```python
from build123d import *

# Parameters (mm, degrees)
BOSS_EXTRUDE1_DEPTH = 300
SKETCH3_R           = 17
SKETCH3_R_2         = 30
CUT_EXTRUDE1_DEPTH  = 1055.907875982
SKETCH4_R           = 90
CUT_EXTRUDE2_DEPTH  = 20
SKETCH5_R           = 17
CUT_EXTRUDE3_DEPTH  = 1051
CHAMFER1_SIZE       = 70
CHAMFER1_SIZE2      = 120
FILLET1_R           = 20


with BuildPart() as part:
    # Sketch2 → Boss-Extrude1 (new body)
    with BuildSketch(Plane(origin=(0, 0, 0), x_dir=(-1, 0, 0), z_dir=(0, 1, 0))):
        Polygon((0, 0), (673.85334868, 0), (673.85334868, 900), (450, 900), (450, 145.843324447), (0, 145.843324447), align=None)
    extrude(amount=BOSS_EXTRUDE1_DEPTH)

    # Sketch3 → Cut-Extrude1 (cut, through all)
    with BuildSketch(Plane.XY.offset(145.843324447)):
        with Locations((-335, 150)):
            Circle(SKETCH3_R)
        with Locations((-228.822978678, 259.933547355)):
            Circle(SKETCH3_R)
        with Locations((-115, 150)):
            Circle(SKETCH3_R)
        with Locations((-225, 40)):
            Circle(SKETCH3_R)
        with Locations((-225, 150)):
            Circle(SKETCH3_R_2)
    extrude(amount=-CUT_EXTRUDE1_DEPTH, mode=Mode.SUBTRACT)

    # Sketch4 → Cut-Extrude2 (cut)
    with BuildSketch(Plane.XY.offset(145.843324447)):
        with Locations((-225, 150)):
            Circle(SKETCH4_R)
    extrude(amount=-CUT_EXTRUDE2_DEPTH, mode=Mode.SUBTRACT)

    # Sketch5 → Cut-Extrude3 (cut, through all)
    with BuildSketch(Plane.YZ.offset(-450)):
        with Locations(Location((75, 713.5, 0), (0, 0, 270))):
            Circle(SKETCH5_R)
        with Locations(Location((225, 713.5, 0), (0, 0, 270))):
            Circle(SKETCH5_R)
        with Locations(Location((75, 332.343324447, 0), (0, 0, 270))):
            Circle(SKETCH5_R)
        with Locations(Location((225, 332.343324447, 0), (0, 0, 270))):
            Circle(SKETCH5_R)
    extrude(amount=-CUT_EXTRUDE3_DEPTH, mode=Mode.SUBTRACT)

    # Chamfer1
    chamfer1_edges = [part.edges().sort_by_distance(p)[0] for p in [
        (-450, 150, 145.843324447),
    ]]
    chamfer1_side = [part.faces().sort_by_distance(p)[0] for p in [
        (-444.591673087, 150, 145.843324447),
    ]]
    chamfer(chamfer1_edges, length=CHAMFER1_SIZE, length2=CHAMFER1_SIZE2, reference=chamfer1_side[0])

    # Fillet1
    fillet1_edges = [part.edges().sort_by_distance(p)[0] for p in [
        (-380, 150, 145.843324447),
        (-450, 150, 265.843324447),
    ]]
    fillet(fillet1_edges, radius=FILLET1_R)


solid = part.part
```
Check sheet for the modelled part. Datum: model origin and axes. Units: mm. A direction names the side the tool comes from. Coordinates: 2 decimals unless noted, no trailing zeros. Loops run counter-clockwise (first coordinate to the right, second up) from the corner with the lowest first, then second, coordinate; pieces in that order, holes last.
1) Sectioned sample at A-A (y = 150). Record the boundary of the cut face in (x, z), and give its area (3 significant figures).
2) Gauge pin test, flat ends, axial feed: pin 1 (8 mm diameter, centred on y = 111, z = 159.5, fed in from +X); pin 2 (20.5 mm diameter, centred on y = 75, z = 332.34, fed in from +X); pin 3 (1.5 mm diameter, centred on y = 185.5, z = 650, fed in from +X). Record the tip position at first contact, or that the pin passes through.
3) Sectioned sample at B-B (x = -335). Record the boundary of the cut face in (y, z), and give its area (3 significant figures).
4) Release check for a two-part mould opening along X. For faces 4 (the face through (0, 148, 74)), 5 (the face through (-337.213, 166.855, 73.943)), 6 (the face through (-482, 0, 356)) record: released by +X, released by -X, zero draft, split by the parting line, or undercut.
5) Access from +Z, -Z, +X, -X, +Y, -Y to the whole of each face (thin tool, end or side, straight path). Record for faces 1 (the face through (-226, 111, 125.843)), 2 (the face through (-563, 148, 900)), 3 (the face through (-450, 148, 590)).
6) Material ranges on probe 1 along Z at (x, y) = (-308, 109); probe 2 along X at (y, z) = (223, 800.5); probe 3 along Z at (x, y) = (-246.5, 195.5), recorded low to high.
7) Sectioned sample at D-D (y = 40). Record the boundary of the cut face in (x, z), and give its area (3 significant figures).
8) Sectioned sample at C-C (z = 713.5). Record the boundary of the cut face in (x, y).
Check sheet entries:
1. outline: (-673.85, 0) - (-352, 0) - (-352, 145.84) - (-368.51, 145.84) arc R20 cw to (-385.79, 155.77) - (-447.28, 261.17) arc R20 cw to (-450, 271.25) - (-450, 900) - (-673.85, 900) - close; (-318, 0) - (-255, 0) - (-255, 125.84) - (-315, 125.84) - (-315, 145.84) - (-318, 145.84) - close; (-195, 0) - (-132, 0) - (-132, 145.84) - (-135, 145.84) - (-135, 125.84) - (-195, 125.84) - close; (-98, 0) - (0, 0) - (0, 145.84) - (-98, 145.84) - close
1. area: 250,000 mm2
2. pin 1: stops at x = -385.63
2. pin 2: passes through
2. pin 3: stops at x = -450
3. outline: (0, 0) - (133, 0) - (133, 145.84) - (0, 145.84) - close; (167, 0) - (300, 0) - (300, 145.84) - (167, 145.84) - close
3. area: 38,800 mm2
4. face 4: released by +X
4. face 5: undercut
4. face 6: zero draft
5. face 1: +Z
5. face 2: +Z, +X, -X, +Y, -Y
5. face 3: +Z, +X, +Y, -Y
6. probe 1: z = 0 to 145.84
6. probe 2: x = -673.85 to -450
6. probe 3: z = 0 to 125.84
7. outline: (-673.85, 0) - (-242, 0) - (-242, 145.84) - (-368.51, 145.84) arc R20 cw to (-385.79, 155.77) - (-447.28, 261.17) arc R20 cw to (-450, 271.25) - (-450, 900) - (-673.85, 900) - close; (-208, 0) - (0, 0) - (0, 145.84) - (-208, 145.84) - close
7. area: 266,000 mm2
8. outline: (-673.85, 0) - (-450, 0) - (-450, 58) - (-673.85, 58) - close; (-673.85, 92) - (-450, 92) - (-450, 208) - (-673.85, 208) - close; (-673.85, 242) - (-450, 242) - (-450, 300) - (-673.85, 300) - close
